Check sheet for the drawn part. Datum: minimum x, y, z corner. Units: mm. Coordinates: 2 decimals unless noted, no trailing zeros. Loops run counter-clockwise (first coordinate to the right, second up) from the corner with the lowest first, then second, coordinate; pieces in that order, holes last. Notation, with made-up numbers: (87, 18.25) - (120, 18.25) arc R21 ccw to (120, 26.25) - close; hole circle Ø11 at (50.5, 53.5). An arc over 180 degrees is marked (long way). Answer as CSV lines item,"result". Start each with the question number.
1. Material ranges on line 1 (Y direction, x = 12.7, z = 4.25) (1 decimal); line 2 (X direction, y = 94.5, z = 5.75); line 3 (Z direction, x = 37, y = 96.5), recorded low to high. Write a range as [from, to].
2. Cross-section at C-C (x = 12.7). Enter the section's corners in (y, z).
3. Gauge pin test, flat ends, axial feed: P1, Ø2, axis at y = 112, z = 2, coming from the +X side; P2, Ø3, axis at x = 81.5, y = 69, coming from the +Z side; P3, Ø3, axis at x = 11, z = 7, coming from the -Y side; P4, Ø4.5, axis at x = 49.53, y = 102.5, coming from the -Z side. Record the tip position at first contact, or that the pin passes through.
4. Cross-section at D-D (y = 120.5). Enter the section's corners in (x, z), plus the area to 3 significant figures.
5. Cross-section at A-A (x = 49.53). Enter the section's corners in (y, z).
6. Cross-section at B-B (z = 2). Enter the section's corners in (x, y), plus the area to 3 significant figures.
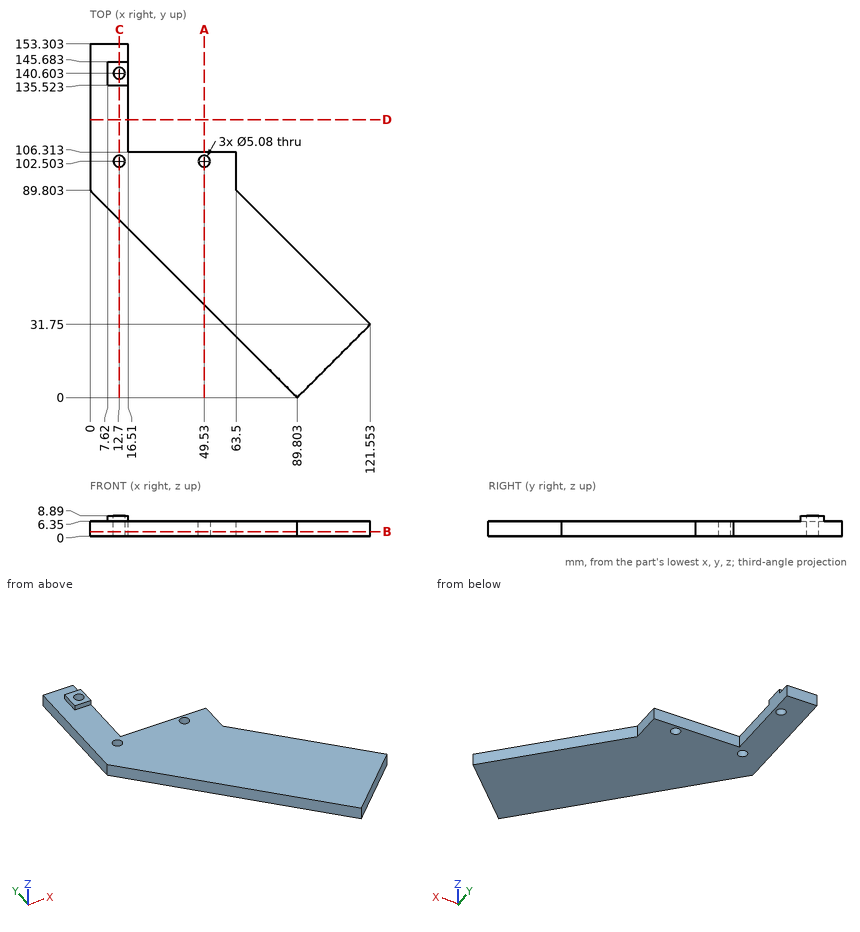
Values follow:
1,line 1,"y = [77.1, 100], [105, 138.1], [143.1, 153.3]"
1,line 2,"x = [0, 63.5]"
1,line 3,"z = [0, 6.35]"
2,outline,"(77.1, 0) - (99.96, 0) - (99.96, 6.35) - (77.1, 6.35) - close; (105.04, 0) - (138.06, 0) - (138.06, 8.89) - (135.52, 8.89) - (135.52, 6.35) - (105.04, 6.35) - close; (143.14, 0) - (153.3, 0) - (153.3, 6.35) - (145.68, 6.35) - (145.68, 8.89) - (143.14, 8.89) - close"
3,P1,"stops at x = 16.51"
3,P2,"stops at z = 6.35"
3,P3,"stops at y = 77.45"
3,P4,"passes through"
4,outline,"(0, 0) - (16.51, 0) - (16.51, 6.35) - (0, 6.35) - close"
4,area,"105 mm²"
5,outline,"(40.27, 0) - (99.96, 0) - (99.96, 6.35) - (40.27, 6.35) - close; (105.04, 0) - (106.31, 0) - (106.31, 6.35) - (105.04, 6.35) - close"
6,outline,"(0, 89.8) - (89.8, 0) - (121.55, 31.75) - (63.5, 89.8) - (63.5, 106.31) - (16.51, 106.31) - (16.51, 153.3) - (0, 153.3) - close; hole circle Ø5.08 at (12.7, 102.5); hole circle Ø5.08 at (12.7, 140.6); hole circle Ø5.08 at (49.53, 102.5)"
6,area,"6,460 mm²"
